Source: CAD feature listing. Evaluate the final solid. Frame: model axes, mm. A direction names the side the tool comes from. Coordinates: 2 decimals unless noted, no trailing zeros. Write each loop counter-clockwise with the first axis right and the second up, starting at its lowest first coordinate (ties: lowest second). Pieces come first, ordered by that corner, then holes. Notation, with made-up numbers: (-12.75, 41) -> (31.25, 41) arc R23 ccw to (31.25, 63) -> close; hole circle Ø9 at (-11.75, 47). An arc over 180 degrees is marked (long way). One line per item, written item: value. Start each with the question number.
1. Section query B-B, the plane x = 0. Output: boundary loops of the cut face in (y, z), and give its area (4 significant figures).
2. Section query C-C, the plane x = 9.5. Output: boundary loops of the cut face in (y, z), and give its area (3 significant figures).
3. Section query A-A, the plane y = -1.5. Output: boundary loops of the cut face in (x, z), and give its area (3 significant figures).
4. Line query: line 1 (Z direction, x = 0, y = -1.7); line 2 (Z direction, x = -3.5, y = -2.7); line 3 (Z direction, x = 9.5, y = -1.85). Output: solid intervals per line, ascending.
5. First-contact query: P1, Ø2.5, axis at x = 0, z = 31.5, coming from the -Y side; P2, Ø4, axis at x = -0.5, z = 31, coming from the +Y side; P3, Ø1, axis at y = -3, z = 30.5, coming from the -X side. Flat tips, straight axial feed; report the tip coordinate or a pass-through.
6. Access query for faces 1 (the flat face through (-0.9, -0.95, 32.4)), 2 (the flat face through (0, -2, -22.5)), 3 (the flat face through (-0.9, -2.45, 32.4)). Directions: +Z, -Z, +X, -X, +Y, -Y. A direction counts if a zero-diameter tool reaches every point of the face in a straight line with its end or side. Return the directions, or none.
7. Section query D-D, the plane x = 13.5. Output: boundary loops of the cut face in (y, z), and give its area (3 significant figures).
8. Mould query, pull axis Z, two halves, no side actions, for faces 4 (the flat face through (13.7, -1.7, 27.7)), 5 (the cylindrical face through (9.305, -1.676, 30.987)), 6 (the flat face through (0, 0, 7)), 7 (the cylindrical face through (-1.11, -1.69, 32.01)). Classes: released by +Z, released by -Z, zero draft, split by the parting line, or undercut.
from build123d import *

# Parameters (mm, degrees)
F1_R     = 1.5
F1_W     = 22
F1_H     = 13
F2_DEPTH = 3.4
F3_W     = 8
F3_H     = 0.95
F4_DEPTH = 8
F5_DEPTH = 8
F6_R     = 5
F7_R     = 5
F8_R     = 5
F9_R     = 5


with BuildPart() as f2:
    # F1 (on Front) → F2 (new body)
    with BuildSketch(Plane.XZ):
        Polygon((15.5, -22.5), (15.5, 22.5), (11, 22.5), (11, 9.5), (-11, 9.5), (-11, 22.5), (-15.5, 22.5), (-15.5, -22.5), align=None)
        Polygon((11, 22.5), (15.5, 22.5), (11, 35.5), (11, 29.5), align=None)
        Polygon((-11, 22.5), (11, 22.5), (11, 29.5), (11, 35.5), (-11, 35.5), align=None)
        with Locations((0, 31)):
            Circle(F1_R, mode=Mode.SUBTRACT)
        with Locations((9.5, 29.5)):
            Circle(F1_R, mode=Mode.SUBTRACT)
        Polygon((-15.5, 22.5), (-11, 22.5), (-11, 35.5), align=None)
        with Locations((0, 16)):
            Rectangle(F1_W, F1_H)
    extrude(amount=F2_DEPTH)

    # F3 (on face) → F4 (cut)
    with BuildSketch(Plane.XY.offset(35.5)):
        with Locations((0, -0.475)):
            Rectangle(F3_W, F3_H)
    extrude(amount=-F4_DEPTH, mode=Mode.SUBTRACT)

    # F3 (on face) → F5 (cut)
    with BuildSketch(Plane.XY.offset(35.5)):
        with Locations((0, -2.925)):
            Rectangle(F3_W, F3_H)
    extrude(amount=-F5_DEPTH, mode=Mode.SUBTRACT)

    # F6
    f6_edges = [f2.edges().sort_by_distance(p)[0] for p in [
        (-11, -1.7, 35.5),
    ]]
    fillet(f6_edges, radius=F6_R)

    # F7
    f7_edges = [f2.edges().sort_by_distance(p)[0] for p in [
        (11, -1.7, 35.5),
    ]]
    fillet(f7_edges, radius=F7_R)

    # F8
    f8_edges = [f2.edges().sort_by_distance(p)[0] for p in [
        (15.5, -1.7, 22.5),
    ]]
    fillet(f8_edges, radius=F8_R)

    # F9
    f9_edges = [f2.edges().sort_by_distance(p)[0] for p in [
        (-15.5, -1.7, 22.5),
    ]]
    fillet(f9_edges, radius=F9_R)


solid = f2.part
Computed values:
1. outline: (-3.4, -22.5) -> (0, -22.5) -> (0, 27.5) -> (-0.95, 27.5) -> (-0.95, 29.5) -> (-2.45, 29.5) -> (-2.45, 27.5) -> (-3.4, 27.5) -> close; (-2.45, 32.5) -> (-0.95, 32.5) -> (-0.95, 35.5) -> (-2.45, 35.5) -> close
1. area: 177.5 mm²
2. outline: (-3.4, -22.5) -> (0, -22.5) -> (0, 28) -> (-3.4, 28) -> close; (-3.4, 31) -> (0, 31) -> (0, 35.06) -> (-3.4, 35.06) -> close
2. area: 185 mm²
3. outline: (-15.5, -22.5) -> (15.5, -22.5) -> (15.5, 21.66) arc R5 ccw to (15.22, 23.29) -> (12.16, 32.14) arc R5 ccw to (7.44, 35.5) -> (-7.44, 35.5) arc R5 ccw to (-12.16, 32.14) -> (-15.22, 23.29) arc R5 ccw to (-15.5, 21.66) -> close; hole circle Ø3 at (0, 31); hole circle Ø3 at (9.5, 29.5)
3. area: 1,720 mm²
4. line 1: z = -22.5 to 29.5, 32.5 to 35.5
4. line 2: z = -22.5 to 27.5
4. line 3: z = -22.5 to 28, 31 to 35.06
5. P1: stops at y = -2.45
5. P2: stops at y = -0.95
5. P3: stops at x = -12.9
6. face 1: +Z, +Y
6. face 2: -Z, +X, -X, +Y, -Y
6. face 3: +Z, -Y
7. outline: (-3.4, -22.5) -> (0, -22.5) -> (0, 28.28) -> (-3.4, 28.28) -> close
7. area: 173 mm²
8. face 4: released by +Z
8. face 5: undercut
8. face 6: zero draft
8. face 7: undercut
